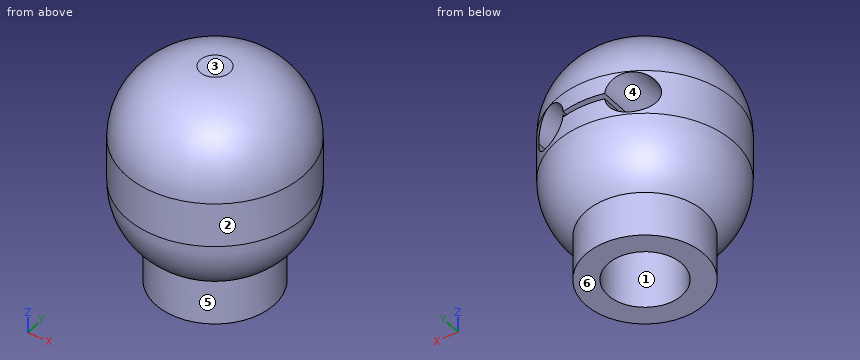
```python
from build123d import *

# Parameters (mm, degrees)
F0_R     = 4
F1_DEPTH = 3
F2_R     = 6
F3_DEPTH = 12
F4_R     = 5
F6_R     = 2.5
F7_DEPTH = 8
F9_DEPTH = 8


# Not quite as in the source:
# - a fillet or chamfer that OpenCascade refuses, or shapes differently, is made with other operations: its cross-section is extruded or revolved along the edge and cut away or added


with BuildPart() as f1:
    # F0 (on Top) → F1 (new body)
    with BuildSketch(Plane.XY):
        Circle(F0_R)
    extrude(amount=F1_DEPTH)

    # F2 (on face) → F3 (join)
    with BuildSketch(Plane.XY.offset(3)):
        Circle(F2_R)
    extrude(amount=F3_DEPTH)

    # F4
    f4_edges = [f1.edges().sort_by_distance(p)[0] for p in [
        (-6, 0, 15),
    ]]
    fillet(f4_edges, radius=F4_R)

    # F5: fillet of radius 5 on 1 edges, made by hand

    # F5_s1 → F5_t2 (revolve, cut)
    with BuildSketch(Plane.XZ):
        with BuildLine():
            ThreePointArc((6, 7), (5.472135955, 4.7639320225), (4, 3))
            Line((4, 3), (6, 3))
            Line((6, 3), (6, 7))
        make_face()
    revolve(axis=Axis((0, 0, 3), (0, 0, 1)), mode=Mode.SUBTRACT)

    # F6 (on face) → F7 (cut)
    with BuildSketch(Plane(origin=(0, 0, 0), x_dir=(1, 0, 0), z_dir=(0, 0, -1))):
        Circle(F6_R)
    extrude(amount=-F7_DEPTH, mode=Mode.SUBTRACT)

    # F8 (on Front) → F9 (cut)
    with BuildSketch(Plane.XZ):
        with BuildLine():
            Line((-1.3463870705, 8.7240217328), (-1.3463870705, 8.3487899899))
            ThreePointArc((-1.3463870705, 8.3487899899), (-1.3369403935, 8.4423866045), (-1.3337867757, 8.5364058614))
            ThreePointArc((-1.3337867757, 8.5364058614), (-1.3369403935, 8.6304251183), (-1.3463870705, 8.7240217328))
        make_face()
        with BuildLine():
            ThreePointArc((-1.3337867757, 8.5364058614), (-1.3369403935, 8.4423866045), (-1.3463870705, 8.3487899899))
            Line((-1.3463870705, 8.3487899899), (1.4683810595, 8.3487899899))
            Line((1.4683810595, 8.3487899899), (1.4683810595, 8.5058610392))
            ThreePointArc((1.4683810595, 8.5058610392), (1.4637016301, 8.6179580539), (1.4683810595, 8.7300550686))
            Line((1.4683810595, 8.7300550686), (-1.3463870705, 8.7300550686))
            Line((-1.3463870705, 8.7300550686), (-1.3463870705, 8.7240217328))
            ThreePointArc((-1.3463870705, 8.7240217328), (-1.3369403935, 8.6304251183), (-1.3337867757, 8.5364058614))
        make_face()
        with BuildLine():
            ThreePointArc((-1.3463870705, 8.7240217328), (-4.1399498979, 8.5364058614), (-1.3463870705, 8.3487899899))
            Line((-1.3463870705, 8.3487899899), (-1.3463870705, 8.7240217328))
        make_face()
        with BuildLine():
            Line((1.4683810595, 8.7300550686), (1.4683810595, 8.5058610392))
            ThreePointArc((1.4683810595, 8.5058610392), (2.864796007, 7.2741313647), (4.1536957416, 8.6179580539))
            ThreePointArc((4.1536957416, 8.6179580539), (2.864796007, 9.9617847432), (1.4683810595, 8.7300550686))
        make_face()
        with BuildLine():
            ThreePointArc((1.4683810595, 8.7300550686), (1.4637016301, 8.6179580539), (1.4683810595, 8.5058610392))
            Line((1.4683810595, 8.5058610392), (1.4683810595, 8.7300550686))
        make_face()
    extrude(amount=-F9_DEPTH, mode=Mode.SUBTRACT)


solid = f1.part
```
Check sheet for the modelled part. Datum: model origin and axes. Units: mm. Face numbers are marked on the shaded views. A direction names the side the tool comes from. Coordinates: 2 decimals unless noted, no trailing zeros. Loops run counter-clockwise (first coordinate to the right, second up) from the corner with the lowest first, then second, coordinate; pieces in that order, holes last. Notation, with made-up numbers: M 9.5,64 L 28.5,64 A18 ccw 28.5,75 Z; hole C -15,15.5 d11. An arc over 180 degrees is marked long. Answer as a JSON object with one key per item and string values.
1. Sectioned sample at B-B on z = 1.5. Record the cut outline in (x, y), and give its area (3 significant figures).
Outcome:
{"outline": "C 0,0 d8; hole C 0,0 d5", "area": "30.6 mm²"}
2. Access from +Z, -Z, +X, -X, +Y, -Y to the whole of each face (thin tool, end or side, straight path). Record for the marked faces 1 and 2.
Outcome:
{"face 1": "-Z", "face 2": "+Z, -Z"}
3. Depth check by flat-ended pin: P1, Ø4, axis at x = 0, y = 0, coming from the -Z side; P2, Ø4, axis at y = -2, z = 11, coming from the +X side; P3, Ø3, axis at y = 0.5, z = 4.5, coming from the +X side. Enter the tip coordinate at first touch or a pass-through.
Outcome:
{"P1": "z = 8", "P2": "x = 6", "P3": "x = 5.89"}
4. Scan lines: L1, parallel to Y at x = 0, z = 2.25; L2, parallel to Z at x = -0.5, y = 1; L3, parallel to Z at x = 2.75, y = 0.5. Record each from-to range of solid material in increasing order. Write a range as from..to.
Outcome:
{"L1": "-4..-2.5, 2.5..4", "L2": "8..8.35, 8.73..15", "L3": "0..7.27, 9.96..14.67"}
5. Sectioned sample at A-A on z = 9.5. Record the cut outline in (x, y), and give its area (3 significant figures).
Outcome:
{"outline": "M -3.76,0 L -3.76,4.68 A6 ccw long 3.82,4.62 L 3.82,0 L 1.79,0 L 1.79,5.73 A6 ccw -1.72,5.75 L -1.72,0 Z", "area": "91.6 mm²"}
6. Release check for a two-part mould opening along Z. For the marked faces 3, 4, 5 and 6 record: pulls with the +Z half, pulls with the -Z half, needs draft (parallel to the pull), parting line crosses it, or undercut.
Outcome:
{"face 3": "pulls with the +Z half", "face 4": "undercut", "face 5": "needs draft", "face 6": "pulls with the -Z half"}
